from build123d import *

# Parameters (mm, degrees)
F0_W     = 914.4
F0_H     = 1524
F1_DEPTH = 609.6
F2_W     = 863.6
F2_H     = 228.6
F3_DEPTH = 584.2
F4_W     = 863.6
F4_H     = 685.8
F5_DEPTH = 584.2


with BuildPart() as f1:
    # F0 (on Right) → F1 (new body)
    with BuildSketch(Plane.YZ):
        Rectangle(F0_W, F0_H)
    extrude(amount=F1_DEPTH)

    # F2 (on face) → F3 (cut)
    with BuildSketch(Plane.YZ.offset(609.6)):
        with Locations((0, 622.3)):
            Rectangle(F2_W, F2_H)
        with Locations((0, 368.3)):
            Rectangle(F2_W, F2_H)
        with Locations((0, 114.3)):
            Rectangle(F2_W, F2_H)
    extrude(amount=-F3_DEPTH, mode=Mode.SUBTRACT)

    # F4 (on face) → F5 (cut)
    with BuildSketch(Plane.YZ.offset(609.6)):
        with Locations((0, -368.3)):
            Rectangle(F4_W, F4_H)
    extrude(amount=-F5_DEPTH, mode=Mode.SUBTRACT)


solid = f1.part
Could you check a few things on this model? Use its own coordinates, in mm. A direction names the side the tool comes from. Coordinates: 2 decimals unless noted, no trailing zeros. Loops run counter-clockwise (first coordinate to the right, second up) from the corner with the lowest first, then second, coordinate; pieces in that order, holes last.
1. I need wall thicknesses on L1, parallel to Z at x = 97, y = -28; L2, parallel to Y at x = 358.5, z = 416.5; L3, parallel to X at y = 62, z = -490.5. Which ranges of each line are inside material? Lowest first, please.
2. Imagine slicing it at A-A (x = 143). Please give me the cut outline in (y, z).
3. Imagine slicing it at B-B (z = -237.5). Please give me the cut outline in (x, y), and give its area (3 significant figures).
4. For P1, Ø6, axis at y = 215.5, z = -420.5, coming from the -X side; P2, Ø8, axis at y = 163.5, z = -280, coming from the +X side, each with a flat end and sliding along its axis, tell me the tip position at first contact or that it passes through.
5. Imagine slicing it at C-C (y = -112.5). Please give me the cut outline in (x, z), and give its area (3 significant figures).
6. We'd pull the mould along Z, two halves only. Please class faces 1 (the face through (25.4, -6, 370)), 2 (the face through (301, -6, 762)), 3 (the face through (609.6, -2, 229)): released by +Z, released by -Z, zero draft, split by the parting line, or undercut.
7. For faces 4 (the face through (322, -6, -711.2)), 5 (the face through (301, -6, -762)), which set-ups out of +Z, -Z, +X, -X, +Y, -Y let a thin tool reach every point of the face, with its end or its side?
Computed values:
1. L1: z = -762 to -711.2, -25.4 to 0, 228.6 to 254, 482.6 to 508, 736.6 to 762
1. L2: y = -457.2 to -431.8, 431.8 to 457.2
1. L3: x = 0 to 25.4
2. outline: (-457.2, -762) - (457.2, -762) - (457.2, 762) - (-457.2, 762) - close; hole (-431.8, -711.2) - (431.8, -711.2) - (431.8, -25.4) - (-431.8, -25.4) - close; hole (-431.8, 0) - (431.8, 0) - (431.8, 228.6) - (-431.8, 228.6) - close; hole (-431.8, 254) - (431.8, 254) - (431.8, 482.6) - (-431.8, 482.6) - close; hole (-431.8, 508) - (431.8, 508) - (431.8, 736.6) - (-431.8, 736.6) - close
3. outline: (0, -457.2) - (609.6, -457.2) - (609.6, -431.8) - (25.4, -431.8) - (25.4, 431.8) - (609.6, 431.8) - (609.6, 457.2) - (0, 457.2) - close
3. area: 52,900 mm2
4. P1: stops at x = 0
4. P2: stops at x = 25.4
5. outline: (0, -762) - (609.6, -762) - (609.6, -711.2) - (25.4, -711.2) - (25.4, -25.4) - (609.6, -25.4) - (609.6, 0) - (25.4, 0) - (25.4, 228.6) - (609.6, 228.6) - (609.6, 254) - (25.4, 254) - (25.4, 482.6) - (609.6, 482.6) - (609.6, 508) - (25.4, 508) - (25.4, 736.6) - (609.6, 736.6) - (609.6, 762) - (0, 762) - close
5. area: 128,000 mm2
6. face 1: undercut
6. face 2: released by +Z
6. face 3: zero draft
7. face 4: +X
7. face 5: -Z, +X, -X, +Y, -Y
